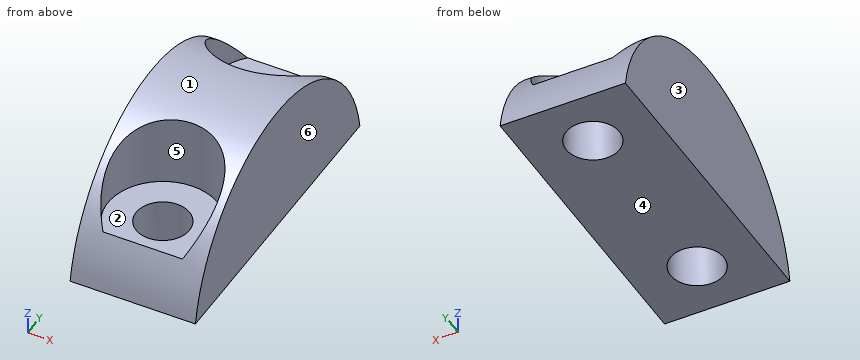
Autodesk Inventor part; units mm, degrees
ref_plane "作業平面1" through (0, 3.6474, 18.0868) normal (0, 0, 1) x (1, 0, 0)
ref_plane "YZ Plane" through (0, 0, 0) normal (1, 0, 0) x (0, 1, 0)
ref_plane "XZ Plane" through (0, 0, 0) normal (0, 1, 0) x (-1, 0, 0)
sketch "スケッチ1" plane through (0, 0, 0) normal (1, 0, 0) x (0, 1, 0)
  circle A0 centre (3.6474, 8.0868) radius 10
  circle A1 centre (3.6474, 8.0868) radius 2.1
  line L0 (2.3974, 9.7742) -> (4.8974, 9.7742)
  line L1 (-4.3526, 14.0868) -> (-4.3526, 2.0868) construction
  line L2 (-1.3526, 16.747) -> (-1.3526, -0.5735) construction
  line L3 (2.3974, 9.7742) -> (13.504, 9.7742)
  line L4 (13.504, 9.7742) -> (-6.2092, 9.7742)
  point P0 (0, 0)
  point P1 (-6.3526, 8.0868)
  dimension "d0" = 20
  dimension "d1" = 4.2
  dimension "d2" = 2.5
  dimension "d3" = 3
  dimension "d4" = 5
extrude "押し出し1" add sketch "スケッチ1" along normal blind 8 contours L3 A1 L4 A0 | L0 A1 picked at (-3.121, 10.5193) picked at (3.6474, 9.9117)
ref_plane "作業平面1" through (0, 3.6474, 18.0868) normal (0, 0, 1) x (1, 0, 0)
sketch "スケッチ2" plane through (0, 3.6474, 18.0868) normal (0, 0, 1) x (1, 0, 0)
  circle A0 centre (4, -6.25) radius 1.7
  line L0 (8, -9.8566) -> (8, 9.8566)
  line L1 (0, -9.8566) -> (0, 9.8566)
  line L2 (0, -1.25) -> (8, -1.25)
  line L3 (8, 0) -> (0, 0)
  circle A1 centre (4, 6.25) radius 1.7
  circle A2 centre (4, -6.25) radius 3.5
  circle A3 centre (4, 6.25) radius 3.5
  point P0 (0, -3.6474)
  dimension "d7" = 3.4
  dimension "d9" = 4
  dimension "d10" = 1.25
  dimension "d11" = 5
  dimension "d14" = 7
  dimension "d15" = 7
extrude "押し出し2" cut sketch "スケッチ2" against normal blind 15 contours A0 | A1
extrude "押し出し3" cut sketch "スケッチ2" against normal blind 5 contours A0 | A2 | A3
properties part number "RZvector-v1-3DP-E-F" material "ABS プラスチック"
Input: part model. Units: mm. Frame: model coordinates. Face numbers are marked on the shaded views. A direction names the side the tool comes from. Coordinates: 2 decimals unless noted, no trailing zeros. Loops run counter-clockwise (first coordinate to the right, second up) from the corner with the lowest first, then second, coordinate; pieces in that order, holes last. Notation, with made-up numbers: (32, 25.25) -> (63, 25.25) arc R24 ccw to (63, 61.25) -> close; hole circle Ø6 at (87, 22). An arc over 180 degrees is marked (long way). One line per item, written item: value.
(1) Ray query, line 1 along Y through (x, z) = (4, 11.25); line 2 along Y through (x, z) = (4, 10.9); line 3 along Z through (x, y) = (3.25, 0.5). Return the intervals inside material, ascending.
Answer below:
line 1: y = -5.84 to -4.3, -0.9 to 8.2, 11.6 to 13.13
line 2: y = -5.95 to -4.3, -0.9 to 8.2, 11.6 to 13.24
line 3: z = 9.77 to 13.09
(2) Cut plane D-D (x = 5). Output: boundary loops of the cut face in (y, z).
Answer below:
outline: (-6.21, 9.77) -> (-3.98, 9.77) -> (-3.98, 13.09) -> (-5.01, 13.09) arc R10 ccw to start; (-1.23, 9.77) -> (8.52, 9.77) -> (8.52, 13.09) -> (6.54, 13.09) -> (6.54, 17.66) arc R10 ccw to (0.75, 17.66) -> (0.75, 13.09) -> (-1.23, 13.09) -> close; (11.27, 9.77) -> (13.5, 9.77) arc R10 ccw to (12.31, 13.09) -> (11.27, 13.09) -> close
(3) Cut plane B-B (y = 11). Output: boundary loops of the cut face in (x, z), then the cut area to 3 significant figures.
Answer below:
outline: (0, 9.77) -> (2.71, 9.77) -> (2.71, 13.09) -> (0.68, 13.09) -> (0.68, 14.86) -> (0, 14.86) -> close; (5.29, 9.77) -> (8, 9.77) -> (8, 14.86) -> (7.32, 14.86) -> (7.32, 13.09) -> (5.29, 13.09) -> close
area: 20.3 mm2
(4) Pin query (flat end, axial travel): pin 1 Ø4.5 at (x, y) = (4, 9.9) entering from +Z; pin 2 Ø1.5 at (x, z) = (4, 16.5) entering from -Y; pin 3 Ø4 at (x, z) = (3, 15) entering from +Y. Return the tip coordinate at first contact, or that it passes through.
Answer below:
pin 1: stops at z = 13.09
pin 2: stops at y = 0.82
pin 3: stops at y = 12.36
(5) Set-up query: the marked faces 1 and 2. Return all of +Z, -Z, +X, -X, +Y, -Y with unobstructed straight access to the full face (end or side cutting, diameter ignored); none if empty.
Answer below:
face 1: +Z, +X, -X
face 2: +Z
(6) Cut plane A-A (x = 4). Output: boundary loops of the cut face in (y, z), then the cut area to 3 significant figures.
Answer below:
outline: (-6.21, 9.77) -> (-4.3, 9.77) -> (-4.3, 13.09) -> (-5.01, 13.09) arc R10 ccw to start; (-0.9, 9.77) -> (8.2, 9.77) -> (8.2, 13.09) -> (6.4, 13.09) -> (6.4, 17.7) arc R10 ccw to (0.9, 17.7) -> (0.9, 13.09) -> (-0.9, 13.09) -> close; (11.6, 9.77) -> (13.5, 9.77) arc R10 ccw to (12.31, 13.09) -> (11.6, 13.09) -> close
area: 66.3 mm2
(7) Cut plane C-C (z = 10.5). Output: boundary loops of the cut face in (x, y).
Answer below:
outline: (0, -6.06) -> (8, -6.06) -> (8, 13.35) -> (0, 13.35) -> close; hole circle Ø3.4 at (4, -2.6); hole circle Ø3.4 at (4, 9.9)
(8) Draft query along X for the marked faces 3, 4, 5 and 6. Return one class per face: pulls with the +X half, pulls with the -X half, needs draft (parallel to the pull), parting line crosses it, or undercut.
Answer below:
face 3: pulls with the -X half
face 4: needs draft
face 5: undercut
face 6: pulls with the +X half
